Part model, mm, in its own coordinate system. Face numbers are marked on the shaded views. A direction names the side the tool comes from. Round coordinates to 2 decimals unless told otherwise and drop trailing zeros. Write each loop counter-clockwise with the first axis right and the second up, starting at its lowest first coordinate (ties: lowest second). Pieces come first, ordered by that corner, then holes. Notation, with made-up numbers: (43, -35) -> (52, -35) arc R18 cw to (52, -9) -> close; hole circle Ø9 at (-11, 63). An arc over 180 degrees is marked (long way). Return JSON: item names as keys, results as strings. Group by question number.
(1) Tool access for the marked faces 1, 2, 3, 4 and 5: list every direction of +Z, -Z, +X, -X, +Y, -Y with a clear straight run to the whole face (end or side of a thin tool).
(2) Drill centre lines: L1, parallel to X at y = 17.65, z = 15; L2, parallel to X at y = 3.25, z = 48; L3, parallel to X at y = 14.25, z = 15. Where is each one in solid material? Low to high. Write a range as from..to.
(3) Saw through at A-A (x = -76.5). List the corners of the cut face in (y, z), plus the area to 3 significant figures.
(4) Saw through at C-C (z = 102.5). State how many separate pieces and enclosed holes the cut face has, plus the area to 3 significant figures.
(5) Saw through at B-B (y = 8). List the corners of the cut face in (x, z), plus the area to 3 significant figures.
(6) Drop flat-ended pins along their axis: pin 1 Ø5 at (x, y) = (17, 5.5) entering from -Z; pin 2 Ø3 at (y, z) = (14.5, 100.5) entering from +X; pin 3 Ø6.5 at (x, z) = (-76.5, 102.5) entering from -Y. Give the stop position or say it passes through.
(7) Mould opens along Z. For the marked faces 6, 7 and 8 say: +Z half, -Z half, draft (parallel to the pull), parting line (faces both ways), or undercut.
from build123d import *

# Parameters (mm, degrees)
SKETCH1_W           = 90
SKETCH1_H           = 22
BOSS_EXTRUDE1_DEPTH = 16
SKETCH2_W           = 119.5
SKETCH2_H           = 18
CUT_EXTRUDE1_DEPTH  = 10
SWEEP5_START        = 10
SWEEP5_DEPTH        = 6
SWEEP5_2_DEPTH      = 10
BOSS_EXTRUDE2_DEPTH = 90
SKETCH12_W          = 8
SKETCH12_H          = 11
SKETCH12_H_2        = 8
SKETCH12_R          = 2
BOSS_EXTRUDE3_DEPTH = 3
SKETCH14_W          = 8
SKETCH14_H          = 8
SKETCH14_R          = 2
SKETCH14_W_2        = 11
BOSS_EXTRUDE4_DEPTH = 4
FILLET1_R           = 2


# Read off the part's stored shape, not the designer's step: Sweep5
with BuildPart() as part:
    # Sketch1 → Boss-Extrude1 (new body)
    with BuildSketch(Plane(origin=(0, 0, 0), x_dir=(1, 0, 0), z_dir=(0, 1, 0))):
        Rectangle(SKETCH1_W, SKETCH1_H)
    extrude(amount=BOSS_EXTRUDE1_DEPTH)

    # Sketch2 → Cut-Extrude1 (cut)
    with BuildSketch(Plane.XZ):
        Rectangle(SKETCH2_W, SKETCH2_H)
    extrude(amount=-CUT_EXTRUDE1_DEPTH, mode=Mode.SUBTRACT)

    # Sweep5 outline → Sweep5 (add)
    with BuildSketch(Plane(origin=(0, 0, 0), x_dir=(1, 0, 0), z_dir=(0, 1, 0)).offset(SWEEP5_START)):
        with BuildLine():
            ThreePointArc((-45, 11), (-64.445436483, 2.945436483), (-72.5, -16.5))
            Line((-72.5, -16.5), (-50.5, -16.5))
            ThreePointArc((-50.5, -16.5), (-48.889087297, -12.610912703), (-45, -11))
            Line((-45, -11), (-45, 11))
        make_face()
    extrude(amount=SWEEP5_DEPTH)

    # Sweep5 2 outline → Sweep5 2 (add)
    with BuildSketch(Plane(origin=(0, 0, 0), x_dir=(1, 0, 0), z_dir=(0, 1, 0))):
        with BuildLine():
            ThreePointArc((-45, 11), (-64.445436483, 2.945436483), (-72.5, -16.5))
            Line((-72.5, -16.5), (-70.5, -16.5))
            ThreePointArc((-70.5, -16.5), (-63.03122292, 1.53122292), (-45, 9))
            Line((-45, 9), (-45, 11))
        make_face()
        with BuildLine():
            ThreePointArc((-45, -9), (-50.303300859, -11.196699141), (-52.5, -16.5))
            Line((-52.5, -16.5), (-50.5, -16.5))
            ThreePointArc((-50.5, -16.5), (-48.889087297, -12.610912703), (-45, -11))
            Line((-45, -11), (-45, -9))
        make_face()
    extrude(amount=SWEEP5_2_DEPTH)

    # Sketch11 → Boss-Extrude2 (add)
    with BuildSketch(Plane.XY.offset(16.5)):
        Polygon((-72.5, 16), (-72.5, 0), (-70.5, 0), (-70.5, 10), (-52.5, 10), (-52.5, 0), (-50.5, 0), (-50.5, 16), align=None)
    extrude(amount=BOSS_EXTRUDE2_DEPTH)

    # Sketch12 → Boss-Extrude3 (add, symmetric)
    # profile 1 of 4: a face of its own
    with BuildSketch(Plane(origin=(0, 16, 0), x_dir=(1, 0, 0), z_dir=(0, 1, 0))):
        with Locations((41, 5.5)):
            Rectangle(SKETCH12_W, SKETCH12_H)
    # profile 2 of 4: a face of its own
    with BuildSketch(Plane(origin=(0, 16, 0), x_dir=(1, 0, 0), z_dir=(0, 1, 0))):
        with Locations((41, -5.5)):
            Rectangle(SKETCH12_W, SKETCH12_H)
    # profile 3 of 4: a face of its own
    with BuildSketch(Plane(origin=(0, 16, 0), x_dir=(1, 0, 0), z_dir=(0, 1, 0))):
        with Locations((41, -15)):
            Rectangle(SKETCH12_W, SKETCH12_H_2)
        with Locations(Location((41, -15, 0), (0, 0, 270))):
            Circle(SKETCH12_R, mode=Mode.SUBTRACT)
    # profile 4 of 4: a face of its own
    with BuildSketch(Plane(origin=(0, 16, 0), x_dir=(1, 0, 0), z_dir=(0, 1, 0))):
        with Locations((41, 15)):
            Rectangle(SKETCH12_W, SKETCH12_H_2)
        with Locations(Location((41, 15, 0), (0, 0, 270))):
            Circle(SKETCH12_R, mode=Mode.SUBTRACT)
    extrude(amount=BOSS_EXTRUDE3_DEPTH, both=True)

    # Sketch14 → Boss-Extrude4 (add)
    # profile 1 of 4: a face of its own
    with BuildSketch(Plane(origin=(0, 16, 0), x_dir=(1, 0, 0), z_dir=(0, 1, 0))):
        with Locations((-76.5, -102.5)):
            Rectangle(SKETCH14_W, SKETCH14_H)
        with Locations(Location((-76.5, -102.5, 0), (0, 0, 270))):
            Circle(SKETCH14_R, mode=Mode.SUBTRACT)
    # profile 2 of 4: a face of its own
    with BuildSketch(Plane(origin=(0, 16, 0), x_dir=(1, 0, 0), z_dir=(0, 1, 0))):
        with Locations((-67, -102.5)):
            Rectangle(SKETCH14_W_2, SKETCH14_H)
    # profile 3 of 4: a face of its own
    with BuildSketch(Plane(origin=(0, 16, 0), x_dir=(1, 0, 0), z_dir=(0, 1, 0))):
        with Locations((-56, -102.5)):
            Rectangle(SKETCH14_W_2, SKETCH14_H)
    # profile 4 of 4: a face of its own
    with BuildSketch(Plane(origin=(0, 16, 0), x_dir=(1, 0, 0), z_dir=(0, 1, 0))):
        with Locations((-46.5, -102.5)):
            Rectangle(SKETCH14_W, SKETCH14_H)
        with Locations(Location((-46.5, -102.5, 0), (0, 0, 270))):
            Circle(SKETCH14_R, mode=Mode.SUBTRACT)
    extrude(amount=-BOSS_EXTRUDE4_DEPTH)

    # Fillet1
    fillet1_edges = [part.edges().sort_by_distance(p)[0] for p in [
        (-50.5, 14, 98.5),
        (-72.5, 12, 102.5),
        (-50.5, 12, 102.5),
        (-72.5, 14, 98.5),
        (37, 16, 0),
        (41, 13, 11),
        (41, 13, -11),
        (37, 14.5, -11),
        (37, 14.5, 11),
    ]]
    fillet(fillet1_edges, radius=FILLET1_R - 0.0001)  # a hair under: the kernel refuses the full size


solid = part.part
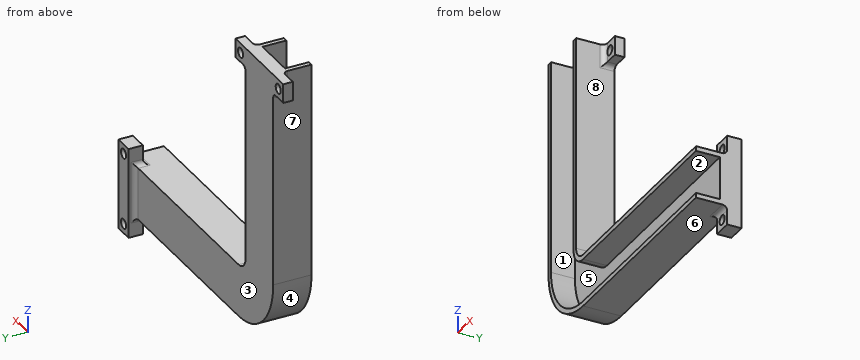
Computed values:
{
 "1": {"face 1": "+Z, -Y", "face 2": "+X, -Y", "face 3": "+Z, -Z, -X, +Y", "face 4": "-Z, -X, +Y, -Y", "face 5": "-Y"},
 "2": {"L1": "37..39, 43..45", "L2": "-72.5..-70.5, -52.5..-50.5", "L3": "-72.46..-50.29, 37..39, 43..45"},
 "3": {"outline": "(12, 98.5) -> (16, 98.5) -> (16, 100.5) -> (12, 100.5) -> close; (12, 104.5) -> (16, 104.5) -> (16, 106.5) -> (12, 106.5) -> close", "area": "16.0 mm2"},
 "4": {"separate pieces": "3", "enclosed holes": "0", "area": "206 mm2"},
 "5": {"outline": "(-72.5, 16.5) arc R27.5 ccw to (-45, -11) -> (45, -11) -> (45, -9) -> (-45, -9) arc R25.5 cw to (-70.5, 16.5) -> (-70.5, 106.5) -> (-72.5, 106.5) -> close; (-52.5, 16.5) arc R7.5 ccw to (-45, 9) -> (45, 9) -> (45, 11) -> (-45, 11) arc R5.5 cw to (-50.5, 16.5) -> (-50.5, 106.5) -> (-52.5, 106.5) -> close", "area": "824 mm2"},
 "6": {"pin 1": "z = -11", "pin 2": "x = -42.5", "pin 3": "y = 11.56"},
 "7": {"face 6": "-Z half", "face 7": "draft", "face 8": "undercut"}
}
